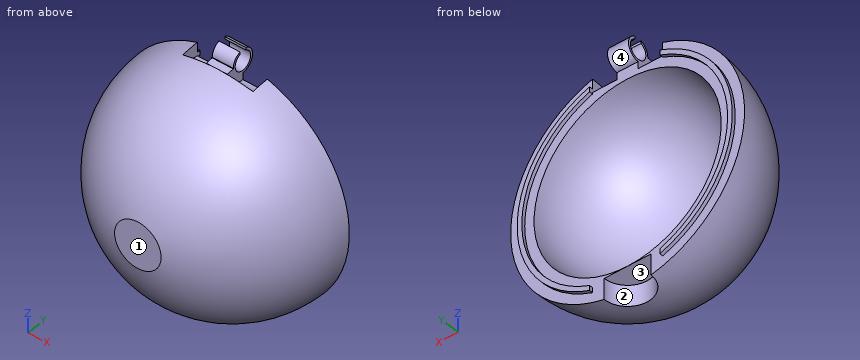
```python
from build123d import *

# Parameters (mm, degrees)
CUT_EXTRUDE1_DEPTH       = 15
CUT_EXTRUDE1_DEPTH_BACK  = 15
SKETCH2_R                = 8
BOSS_EXTRUDE1_DEPTH      = 4.5
BOSS_EXTRUDE1_DEPTH_BACK = 4.5
SKETCH3_R                = 5
SKETCH3_R_2              = 4
BOSS_EXTRUDE2_DEPTH      = 4.5
BOSS_EXTRUDE2_DEPTH_BACK = 4.5
SKETCH5_R                = 10
CUT_EXTRUDE2_DEPTH       = 10
BOSS_EXTRUDE3_DEPTH      = 1.5
BOSS_EXTRUDE6_DEPTH      = 4.5
BOSS_EXTRUDE6_DEPTH_BACK = 4.5
CUT_EXTRUDE3_DEPTH       = 4.5
CUT_EXTRUDE3_DEPTH_BACK  = 4.5
SKETCH11_W               = 10
SKETCH11_H               = 3
SKETCH12_R               = 10
CUT_EXTRUDE4_DEPTH       = 1


with BuildPart() as part:
    # Sketch1 → Revolve1 (revolve)
    with BuildSketch(Plane(origin=(0, 0, 0), x_dir=(0, 0, -1), z_dir=(1, 0, 0))):
        with BuildLine():
            Line((0, -40), (0, -50))
            ThreePointArc((0, -50), (35.355339059, -35.355339059), (50, 0))
            Line((50, 0), (40, 0))
            ThreePointArc((40, 0), (28.284271247, -28.284271247), (0, -40))
        make_face()
    revolve(axis=Axis((0, 58.068573396, 0), (0, -1, 0)))

    # Sketch2 → Cut-Extrude1 (cut, two sides: drawn at the far end of the back side and taken through both)
    with BuildSketch(Plane(origin=(0, 0, 0), x_dir=(0, 0, -1), z_dir=(1, 0, 0)).offset(-CUT_EXTRUDE1_DEPTH_BACK)):
        with Locations((-50, 0)):
            Circle(SKETCH2_R)
    extrude(amount=CUT_EXTRUDE1_DEPTH + CUT_EXTRUDE1_DEPTH_BACK, mode=Mode.SUBTRACT)



with BuildPart() as body_2:
    # Sketch3 → Boss-Extrude1 (new, two sides: drawn at the far end of the back side and taken through both)
    with BuildSketch(Plane(origin=(0, 0, 0), x_dir=(0, 0, -1), z_dir=(1, 0, 0)).offset(-BOSS_EXTRUDE1_DEPTH_BACK)):
        with Locations((-50, 0)):
            Circle(SKETCH3_R)
        with Locations((-50, 0)):
            Circle(SKETCH3_R_2, mode=Mode.SUBTRACT)
    extrude(amount=BOSS_EXTRUDE1_DEPTH + BOSS_EXTRUDE1_DEPTH_BACK)


with BuildPart() as part_1:
    add(part.part)

    add(body_2.part)  # Boss-Extrude2 merges body 2
    # Sketch4 → Boss-Extrude2 (add, two sides: drawn at the far end of the back side and taken through both)
    with BuildSketch(Plane(origin=(0, 0, 0), x_dir=(0, 0, -1), z_dir=(1, 0, 0)).offset(-BOSS_EXTRUDE2_DEPTH_BACK)):
        with BuildLine():
            Line((-46, 0), (-40, 0))
            Line((-40, 0), (-40, -5))
            Line((-40, -5), (-50, -5))
            Line((-50, -5), (-50, -4))
            ThreePointArc((-50, -4), (-47.171572875, -2.828427125), (-46, 0))
        make_face()
    extrude(amount=BOSS_EXTRUDE2_DEPTH + BOSS_EXTRUDE2_DEPTH_BACK)

    # Sketch5 → Cut-Extrude2 (cut)
    with BuildSketch(Plane.XY.offset(-50)):
        Circle(SKETCH5_R)
    extrude(amount=CUT_EXTRUDE2_DEPTH, mode=Mode.SUBTRACT)

    # Sketch6 → Boss-Extrude3 (add)
    with BuildSketch(Plane(origin=(0, 0, 0), x_dir=(1, 0, 0), z_dir=(0, 1, 0))):
        with BuildLine():
            Line((-15, 43.48562981), (-15, 41.36423576))
            ThreePointArc((-15, 41.36423576), (-44, 0), (-15, -41.36423576))
            Line((-15, -41.36423576), (-15, -43.48562981))
            ThreePointArc((-15, -43.48562981), (-46, 0), (-15, 43.48562981))
        make_face()
        with BuildLine():
            Line((15, 43.48562981), (15, 41.36423576))
            ThreePointArc((15, 41.36423576), (44, 0), (15, -41.36423576))
            Line((15, -41.36423576), (15, -43.48562981))
            ThreePointArc((15, -43.48562981), (46, 0), (15, 43.48562981))
        make_face()
    extrude(amount=BOSS_EXTRUDE3_DEPTH)

    # Sketch10 → Boss-Extrude6 (add, two sides: drawn at the far end of the back side and taken through both)
    with BuildSketch(Plane(origin=(0, 0, 0), x_dir=(0, 0, -1), z_dir=(1, 0, 0)).offset(-BOSS_EXTRUDE6_DEPTH_BACK)):
        with BuildLine():
            Line((-49.749371855, -5), (-40, -5))
            Line((-40, -5), (-40, -8))
            Line((-40, -8), (-49.355850717, -8))
            ThreePointArc((-49.355850717, -8), (-49.57530923, -6.502977374), (-49.749371855, -5))
        make_face()
    extrude(amount=BOSS_EXTRUDE6_DEPTH + BOSS_EXTRUDE6_DEPTH_BACK)

    # Sketch11 → Cut-Extrude3 (cut, two sides: drawn at the far end of the back side and taken through both)
    with BuildSketch(Plane(origin=(0, 0, 0), x_dir=(0, 0, -1), z_dir=(1, 0, 0)).offset(-CUT_EXTRUDE3_DEPTH_BACK)):
        with Locations((-55, 0)):
            Rectangle(SKETCH11_W, SKETCH11_H)
    extrude(amount=CUT_EXTRUDE3_DEPTH + CUT_EXTRUDE3_DEPTH_BACK, mode=Mode.SUBTRACT)

    # Sketch12 → Cut-Extrude4 (cut)
    with BuildSketch(Plane(origin=(0, -50, 0), x_dir=(1, 0, 0), z_dir=(0, 1, 0))):
        Circle(SKETCH12_R)
    extrude(amount=CUT_EXTRUDE4_DEPTH, mode=Mode.SUBTRACT)


solid = part_1.part
```
The listing builds one solid part. Answer for the finished solid, in the listing's coordinates (mm). Face numbers are marked on the shaded views. A direction names the side the tool comes from. Give positions to 0.01 mm unless a question says otherwise; leave off trailing zeros. Loops run counter-clockwise (first coordinate to the right, second up) from the corner with the lowest first, then second, coordinate; pieces in that order, holes last. Notation, with made-up numbers: (42, 40.5) - (65, 40.5) arc R28 cw to (65, 71.5) - close; hole circle Ø4 at (20.25, 83.25). An arc over 180 degrees is marked (long way). Return JSON: item names as keys, results as strings. Group by question number.
1. Which of the six approach directions +Z, -Z, +X, -X, +Y, -Y give full straight-line access (tool end or side, diameter ignored) to the marked faces 3 and 4?
2. Straight lines are drawn through the part: line 1 (Y direction, x = 0.5, z = 50); line 2 (Z direction, x = -26, y = -20); line 3 (X direction, y = -0.5, z = -6.5). For each, find the intervals that lie inside material, in ascending order. Write a range as [from, to].
3. Determine the mould class of the marked faces 1 and 2 for opening direction X: pulls with the +X half, pulls with the -X half, needs draft (parallel to the pull), parting line crosses it, or undercut.
4. Find section A-A (z = 12.5). Write down the section's boundary in (x, y).
5. Find section C-C (y = -26.5). Write down the section's boundary in (x, z), then the cut area to 3 significant figures.
6. Given pin 1 Ø9.5 at (x, z) = (35.5, -18) entering from +Y; pin 2 Ø5 at (y, z) = (-5, 43) entering from +X; pin 3 Ø0.8 at (y, z) = (1, -42) entering from -X, each flat-ended and moving along its own axis, determine where each tip first touches the part or whether it passes through.
7. Find section B-B (x = -33.5). Write down the section's boundary in (y, z), then the cut area to 3 significant figures.
Verdict:
{
 "1": {"face 3": "-Z, +Y", "face 4": "+X, -X, +Y"},
 "2": {"line 1": "y = [-5, -4], [4, 5]", "line 2": "z = [-37.74, -22.89], [22.89, 37.74]", "line 3": "x = [-49.57, -39.47], [39.47, 49.57]"},
 "3": {"face 1": "needs draft", "face 2": "undercut"},
 "4": {"outline": "(-48.41, 0) arc R48.41 ccw to (48.41, 0) - (44.27, 0) - (44.27, 1.5) - (42.19, 1.5) - (42.19, 0) - (38, 0) arc R38 cw to (-38, 0) - (-42.19, 0) - (-42.19, 1.5) - (-44.27, 1.5) - (-44.27, 0) - close"},
 "5": {"outline": "circle Ø84.8 at (0, 0); hole circle Ø59.92 at (0, 0)", "area": "2,830 mm^2"},
 "6": {"pin 1": "stops at y = 1.5", "pin 2": "stops at x = 28.92", "pin 3": "stops at x = -19.63"},
 "7": {"outline": "(0, -37.12) - (0, -31.52) - (1.5, -31.52) - (1.5, -28.53) - (0, -28.53) - (0, -21.86) arc R21.86 cw to (0, 21.86) - (0, 28.53) - (1.5, 28.53) - (1.5, 31.52) - (0, 31.52) - (0, 37.12) arc R37.12 ccw to start", "area": "1,420 mm^2"}
}
